```python
from build123d import *

# Parameters (mm, degrees)
F1_DEPTH = 6.35
F2_R     = 31.75
F2_R_2   = 25.4
F3_DEPTH = 50.8
F5_DEPTH = 127
F7_R     = 3.3782
F8_DEPTH = 127


with BuildPart() as f1:
    # F0 (on Front) → F1 (new body)
    with BuildSketch(Plane.XZ):
        with BuildLine():
            ThreePointArc((27.703595981, -26.1557024322), (35.4056281322, -14.0730770112), (38.1, 0))
            ThreePointArc((38.1, 0), (35.4056281322, 14.0730770112), (27.703595981, 26.1557024322))
            ThreePointArc((27.703595981, 26.1557024322), (0, 38.1), (-27.703595981, 26.1557024322))
            ThreePointArc((-27.703595981, 26.1557024322), (-38.1, 0), (-27.703595981, -26.1557024322))
            ThreePointArc((-27.703595981, -26.1557024322), (0, -38.1), (27.703595981, -26.1557024322))
        make_face()
        with BuildLine():
            ThreePointArc((27.703595981, 26.1557024322), (35.4056281322, 14.0730770112), (38.1, 0))
            ThreePointArc((38.1, 0), (35.4056281322, -14.0730770112), (27.703595981, -26.1557024322))
            Line((27.703595981, -26.1557024322), (50.3400329984, -2.1796418694))
            ThreePointArc((50.3400329984, -2.1796418694), (46.8586435824, -2.950469011), (44.8564, 0))
            ThreePointArc((44.8564, 0), (46.8586435824, 2.950469011), (50.3400329984, 2.1796418694))
            Line((50.3400329984, 2.1796418694), (27.703595981, 26.1557024322))
        make_face()
        with BuildLine():
            ThreePointArc((-27.703595981, -26.1557024322), (-38.1, 0), (-27.703595981, 26.1557024322))
            Line((-27.703595981, 26.1557024322), (-50.3400329984, 2.1796418694))
            ThreePointArc((-50.3400329984, 2.1796418694), (-46.8586435824, 2.950469011), (-44.8564, 0))
            ThreePointArc((-44.8564, 0), (-46.8586435824, -2.950469011), (-50.3400329984, -2.1796418694))
            Line((-50.3400329984, -2.1796418694), (-27.703595981, -26.1557024322))
        make_face()
        with BuildLine():
            ThreePointArc((51.2064, 0), (50.981869011, 1.1727564176), (50.3400329984, 2.1796418694))
            ThreePointArc((50.3400329984, 2.1796418694), (46.8586435824, 2.950469011), (44.8564, 0))
            ThreePointArc((44.8564, 0), (46.8586435824, -2.950469011), (50.3400329984, -2.1796418694))
            ThreePointArc((50.3400329984, -2.1796418694), (50.981869011, -1.1727564176), (51.2064, 0))
        make_face()
        with BuildLine():
            ThreePointArc((-44.8564, 0), (-46.8586435824, 2.950469011), (-50.3400329984, 2.1796418694))
            ThreePointArc((-50.3400329984, 2.1796418694), (-51.2064, 0), (-50.3400329984, -2.1796418694))
            ThreePointArc((-50.3400329984, -2.1796418694), (-46.8586435824, -2.950469011), (-44.8564, 0))
        make_face()
    extrude(amount=F1_DEPTH)

    # F2 (on Front) → F3 (join)
    with BuildSketch(Plane.XZ):
        Circle(F2_R)
        Circle(F2_R_2, mode=Mode.SUBTRACT)
    extrude(amount=F3_DEPTH)

    # F5 (cut): a face of the model
    f5_faces = [f1.faces().sort_by_distance(p)[0] for p in [
        (0, -6.35, 0),
    ]]
    extrude(f5_faces, amount=-F5_DEPTH, mode=Mode.SUBTRACT)

    # F7 (on offset) → F8 (cut)
    with BuildSketch(Plane.XZ.offset(127)):
        with Locations((-41.4782, 0)):
            Circle(F7_R)
        with Locations((41.4782, 0)):
            Circle(F7_R)
    extrude(amount=-F8_DEPTH, mode=Mode.SUBTRACT)


solid = f1.part
```
Geometry: final body of the model. Coordinates: model frame, mm. A direction names the side the tool comes from. Coordinates: 2 decimals unless noted, no trailing zeros. Order: outer loops, then holes, each group sorted by start corner. A loop starts at its lowest first (then second) coordinate and runs counter-clockwise, first axis right, second up. Notation, with made-up numbers: M 77,-26.75 L 103,-26.75 A23 ccw 103,-16.75 Z; hole C 6.5,87.5 d10. An arc over 180 degrees is marked long. Answer in a Markdown table with one row per item. Add a question column.
Q1. Section query B-B on y = -4. Return the cut outline in (x, z) (3 decimals), and give its area (3 significant figures).
Q2. Mould query, pull axis X, two halves, no side actions, for faces 3 (the cylindrical face through (38.1, -3.2, 0.1)), 4 (the flat face through (-27, -6.35, 17)), 5 (the cylindrical face through (-0.434, -3.131, -38.098)). Classes: released by +X, released by -X, zero draft, split by the parting line, or undercut.
Q3. Contact query for flat-ended pins moving along their axis: P1, Ø5, axis at y = -34.5, z = -20, coming from the -X side; P2, Ø1, axis at x = 24.5, y = -7, coming from the -Z side; P3, Ø5, axis at y = -27, z = -17, coming from the -X side. Output: stop coordinate, or through.
Q4. Line query: L1, parallel to Z at x = 0, y = -37.5; L2, parallel to Y at x = -32, z = 6; L3, parallel to X at y = -26, z = -1.5. Output: solid intervals per line, ascending.
Q5. Section query C-C on z = -6.5. Return the cut outline in (x, y), and give its area (3 significant figures).
Q6. Reachability of faces 1 (the cylindrical face through (-44.853, -3.219, 0.149)), 2 (the cylindrical face through (-6.883, -28.264, -30.995)) from +Z, -Z, +X, -X, +Y, -Y: full face, straight path, thin tool, end or side. Return the list, or none.
Q7. Section query D-D on y = -33.5. Return the cut outline in (x, z).
Q8. Section query A-A on x = 0. Return the cut outline in (y, z).
Completed:
| question | item | result |
|---|---|---|
| 1 | outline | M -50.34,-2.18 L -27.704,-26.156 A38.1 ccw 27.704,-26.156 L 50.34,-2.18 A3.175 ccw 50.34,2.18 L 27.704,26.156 A38.1 ccw -27.704,26.156 L -50.34,2.18 A3.175 ccw Z; hole C -41.478,0 d6.756; hole C 0,0 d50.8; hole C 41.478,0 d6.756 |
| 1 | area | 3,000 mm2 |
| 2 | face 3 | undercut |
| 2 | face 4 | zero draft |
| 2 | face 5 | split by the parting line |
| 3 | P1 | stops at x = -26.49 |
| 3 | P2 | stops at z = -20.79 |
| 3 | P3 | stops at x = -28.25 |
| 4 | L1 | z = -31.75 to -25.4, 25.4 to 31.75 |
| 4 | L2 | y = -6.35 to 0 |
| 4 | L3 | x = -31.71 to -25.36, 25.36 to 31.71 |
| 5 | outline | M -46.26,-6.35 L -31.08,-6.35 L -31.08,-50.8 L -24.55,-50.8 L -24.55,0 L -46.26,0 Z; M 24.55,-50.8 L 31.08,-50.8 L 31.08,-6.35 L 46.26,-6.35 L 46.26,0 L 24.55,0 Z |
| 5 | area | 856 mm2 |
| 6 | face 1 | +Y, -Y |
| 6 | face 2 | -Y |
| 7 | outline | C 0,0 d63.5; hole C 0,0 d50.8 |
| 8 | outline | M -50.8,-31.75 L -6.35,-31.75 L -6.35,-38.1 L 0,-38.1 L 0,-25.4 L -50.8,-25.4 Z; M -50.8,25.4 L 0,25.4 L 0,38.1 L -6.35,38.1 L -6.35,31.75 L -50.8,31.75 Z |
